Verification items for the finished model (mm, model axes). A direction names the side the tool comes from. Coordinates: 2 decimals unless noted, no trailing zeros. Write each loop counter-clockwise with the first axis right and the second up, starting at its lowest first coordinate (ties: lowest second). Pieces come first, ordered by that corner, then holes. Notation, with made-up numbers: (22, 39.25) -> (62, 39.25) arc R24 ccw to (62, 69.25) -> close; hole circle Ø1 at (-3, -40). An arc over 180 degrees is marked (long way). Answer in a Markdown table with one row per item.
```python
from build123d import *

# Parameters (mm, degrees)
SKETCH_1_W          = 40
SKETCH_1_H          = 55
EXTRUDE_1_DEPTH     = 20
SKETCH_2_R          = 8.05
CUT_EXTRUDE_1_DEPTH = 20
SKETCH_3_W          = 40
SKETCH_3_H          = 20
EXTRUDE_2_DEPTH     = 32.5
SKETCH_6_W          = 15.4
SKETCH_6_H          = 15.4
CUT_EXTRUDE_4_DEPTH = 1000
SKETCH_4_R          = 1.65
CUT_EXTRUDE_2_DEPTH = 40
SKETCH_5_W          = 5
SKETCH_5_H          = 5
CUT_EXTRUDE_3_DEPTH = 6
FILLET_1_R          = 2
SKETCH_7_W          = 47.564048478
SKETCH_7_H          = 11.463166905
CUT_EXTRUDE_5_DEPTH = 100
SKETCH_8_R          = 1.65
CUT_EXTRUDE_6_DEPTH = 1000


with BuildPart() as part:
    # 草图1 → 凸台-拉伸1 (new body)
    with BuildSketch(Plane.XY):
        Rectangle(SKETCH_1_W, SKETCH_1_H)
    extrude(amount=EXTRUDE_1_DEPTH)

    # 草图2 → 切除-拉伸1 (cut)
    with BuildSketch(Plane.XY.offset(20)):
        with Locations((0, 10.5)):
            Circle(SKETCH_2_R)
    extrude(amount=-CUT_EXTRUDE_1_DEPTH, mode=Mode.SUBTRACT)

    # 草图3 → 凸台-拉伸2 (add)
    with BuildSketch(Plane.XZ.offset(27.5)):
        with Locations((0, 10)):
            Rectangle(SKETCH_3_W, SKETCH_3_H)
    extrude(amount=EXTRUDE_2_DEPTH)

    # 草图6 → 切除-拉伸4 (cut)
    with BuildSketch(Plane.XY.offset(20)):
        with Locations((0, -25)):
            Rectangle(SKETCH_6_W, SKETCH_6_H)
    extrude(amount=-CUT_EXTRUDE_4_DEPTH, mode=Mode.SUBTRACT)

    # 草图4 → 切除-拉伸2 (cut)
    with BuildSketch(Plane.XY.offset(20)):
        with Locations((4.5, -42.7)):
            Circle(SKETCH_4_R)
        with Locations((-4.5, -42.7)):
            Circle(SKETCH_4_R)
    extrude(amount=-CUT_EXTRUDE_2_DEPTH, mode=Mode.SUBTRACT)

    # 草图5 → 切除-拉伸3 (cut)
    with BuildSketch(Plane.XZ.offset(60)):
        with Locations((0, 12)):
            Rectangle(SKETCH_5_W, SKETCH_5_H)
    extrude(amount=-CUT_EXTRUDE_3_DEPTH, mode=Mode.SUBTRACT)

    # 圆角1
    fillet_1_edges = [part.edges().sort_by_distance(p)[0] for p in [
        (-20, 27.5, 10),
        (20, 27.5, 10),
    ]]
    fillet(fillet_1_edges, radius=FILLET_1_R)

    # 草图7 → 切除-拉伸5 (cut)
    with BuildSketch(Plane.XY.offset(20)):
        with Locations((0, -55.731583453)):
            Rectangle(SKETCH_7_W, SKETCH_7_H)
    extrude(amount=-CUT_EXTRUDE_5_DEPTH, mode=Mode.SUBTRACT)

    # 草图8 → 切除-拉伸6 (cut)
    with BuildSketch(Plane(origin=(20, 0, 0), x_dir=(0, 0, -1), z_dir=(1, 0, 0))):
        with Locations((-10, -25)):
            Circle(SKETCH_8_R)
    extrude(amount=-CUT_EXTRUDE_6_DEPTH, mode=Mode.SUBTRACT)


solid = part.part
```
1. Depth check by flat-ended pin: P1, Ø8, axis at x = -3.5, y = 10, coming from the -Z side. Enter the tip coordinate at first touch or a pass-through.
Geometry says:
| item | result |
|---|---|
| P1 | through |
2. Thickness scan on line 1 (Y direction, x = 0, z = 16.25); line 2 (X direction, y = -23, z = 18.5); line 3 (Y direction, x = -2, z = 6.75). Record the ranges inside material, lowest first. Write a range as from..to.
Geometry says:
| item | result |
|---|---|
| line 1 | -50..-32.7, -17.3..2.45, 18.55..27.5 |
| line 2 | -20..-7.7, 7.7..20 |
| line 3 | -50..-32.7, -17.3..2.7, 18.3..27.5 |
3. Section check A-A, the plane z = 10. Record the boundary of the cut face in (x, y).
Geometry says:
| item | result |
|---|---|
| outline | (-20, -50) -> (20, -50) -> (20, -26.65) -> (7.7, -26.65) -> (7.7, -32.7) -> (-7.7, -32.7) -> (-7.7, -26.65) -> (-20, -26.65) -> close; (-20, -23.35) -> (-7.7, -23.35) -> (-7.7, -17.3) -> (7.7, -17.3) -> (7.7, -23.35) -> (20, -23.35) -> (20, 25.5) arc R2 ccw to (18, 27.5) -> (-18, 27.5) arc R2 ccw to (-20, 25.5) -> close; hole circle Ø16.1 at (0, 10.5); hole circle Ø3.3 at (-4.5, -42.7); hole circle Ø3.3 at (4.5, -42.7) |
4. Section check B-B, the plane y = -25. Record the boundary of the cut face in (x, z).
Geometry says:
| item | result |
|---|---|
| outline | (-20, 0) -> (-7.7, 0) -> (-7.7, 8.35) -> (-20, 8.35) -> close; (-20, 11.65) -> (-7.7, 11.65) -> (-7.7, 20) -> (-20, 20) -> close; (7.7, 0) -> (20, 0) -> (20, 8.35) -> (7.7, 8.35) -> close; (7.7, 11.65) -> (20, 11.65) -> (20, 20) -> (7.7, 20) -> close |
5. Mould release check, pull along Y, two halves, no side actions. Record for faces 3 (the cylindrical face through (19.4, 26.93, 10.14)), 4 (the flat face through (-7.7, -27, 10)), 5 (the flat face through (20, -12, 10)): released by +Y, released by -Y, zero draft, split by the parting line, or undercut.
Geometry says:
| item | result |
|---|---|
| face 3 | released by +Y |
| face 4 | undercut |
| face 5 | zero draft |
6. Section check D-D, the plane z = 18.75. Record the boundary of the cut face in (x, y).
Geometry says:
| item | result |
|---|---|
| outline | (-20, -50) -> (20, -50) -> (20, 25.5) arc R2 ccw to (18, 27.5) -> (-18, 27.5) arc R2 ccw to (-20, 25.5) -> close; hole circle Ø16.1 at (0, 10.5); hole (-7.7, -32.7) -> (7.7, -32.7) -> (7.7, -17.3) -> (-7.7, -17.3) -> close; hole circle Ø3.3 at (-4.5, -42.7); hole circle Ø3.3 at (4.5, -42.7) |
7. Tool access check on faces 1 (the flat face through (0, -32.7, 10)), 2 (the flat face through (0, 27.5, 10)). Record the directions out of +Z, -Z, +X, -X, +Y, -Y that give a thin tool (end or side, any length) a straight path to the whole face; none if there is none.
Geometry says:
| item | result |
|---|---|
| face 1 | +Z, -Z |
| face 2 | +Z, -Z, +X, -X, +Y |
8. Section check C-C, the plane y = 10.5. Record the boundary of the cut face in (x, z), plus the area to 3 significant figures.
Geometry says:
| item | result |
|---|---|
| outline | (-20, 0) -> (-8.05, 0) -> (-8.05, 20) -> (-20, 20) -> close; (8.05, 0) -> (20, 0) -> (20, 20) -> (8.05, 20) -> close |
| area | 478 mm^2 |
